Autodesk Inventor part; units mm, degrees
ref_plane "YZ Plane" through (0, 0, 0) normal (1, 0, 0) x (0, 1, 0)
ref_plane "XZ Plane" through (0, 0, 0) normal (0, 1, 0) x (-1, 0, 0)
ref_plane "XY Plane" through (0, 0, 0) normal (0, 0, 1) x (1, 0, 0)
sketch "Skizze1" plane through (0, 0, 0) normal (0, 0, 1) x (1, 0, 0)
  circle A0 centre (0, 0) radius 20
  dimension "d0" = 40
extrude "Extrusion1" add sketch "Skizze1" along normal blind 1
sketch "Skizze2" plane through (0, 0, 1) normal (0, 0, 1) x (1, 0, 0)
  circle A0 centre (0, 0) radius 20
  circle A1 centre (0, 0) radius 17
  dimension "d3" = 34
extrude "Extrusion2" add sketch "Skizze2" along normal blind 10 contours A1
sketch "Skizze3" plane through (0, 0, 11) normal (0, 0, 1) x (1, 0, 0)
  circle A0 centre (0, 0) radius 17
  circle A1 centre (0, 0) radius 20
  dimension "d6" = 40
extrude "Extrusion3" add sketch "Skizze3" along normal blind 1 contours A0 | A1
sketch "Skizze6" plane through (0, 0, 12) normal (0, 0, 1) x (1, 0, 0)
  circle A0 centre (0, 0) radius 20
  circle A1 centre (0, 0) radius 5.1
  dimension "d16" = 10.2
extrude "Extrusion6" cut sketch "Skizze6" against normal through all contours A1
properties part number "Motorstange" material "PC/ABS-Kunststoff"
Model file for the job. Use its own axes, mm. A direction names the side the tool comes from. Coordinates: 2 decimals unless noted, no trailing zeros. Loops run counter-clockwise (first coordinate to the right, second up) from the corner with the lowest first, then second, coordinate; pieces in that order, holes last. Notation, with made-up numbers: (-6.5, 15) -> (36.5, 15) arc R25 cw to (36.5, 42) -> close; hole circle Ø1 at (14, 77). An arc over 180 degrees is marked (long way). Answer as a JSON object with one key per item and string values.
Q1. Cut at C-C (y = 15). List the corners of the cut face in (x, z), and give its area (3 significant figures).
Report:
{"outline": "(-13.23, 0) -> (13.23, 0) -> (13.23, 1) -> (8, 1) -> (8, 11) -> (13.23, 11) -> (13.23, 12) -> (-13.23, 12) -> (-13.23, 11) -> (-8, 11) -> (-8, 1) -> (-13.23, 1) -> close", "area": "213 mm2"}
Q2. 3-axis set-ups, long thin cutter, end or side, ignore diameter. For faces 1 (the cylindrical face through (-4.336, 19.524, 0.493)), 2 (the flat face through (-9, -15, 1)): which of +Z, -Z, +X, -X, +Y, -Y reach the whole face in a straight line?
Report:
{"face 1": "+Z, -Z", "face 2": "none"}
Q3. Flat gauge pin, fed straight in: P1, Ø6, axis at x = -2.5, z = 7.5, coming from the +Y side. Where does the tip first touch, or does it go through?
Report:
{"P1": "stops at y = 17"}
Q4. Pull direction Z, two halves, no side cores. Call faces 3 (the cylindrical face through (2.4, -4.5, 6.1)), 4 (the cylindrical face through (9.139, -14.334, 5.93)), 5 (the flat face through (4, -4, 12)): released by +Z, released by -Z, zero draft, split by the parting line, or undercut.
Report:
{"face 3": "zero draft", "face 4": "undercut", "face 5": "released by +Z"}
Q5. Probe probe 1 along Y at (x, z) = (0, 9.75); probe 2 along Z at (x, y) = (15, 10); probe 3 along Y at (x, z) = (3, 9.5). List the from-to ranges inside material, lowest first.
Report:
{"probe 1": "y = -17 to -5.1, 5.1 to 17", "probe 2": "z = 0 to 1, 11 to 12", "probe 3": "y = -16.73 to -4.12, 4.12 to 16.73"}
Q6. Cut at A-A (x = 0). List the corners of the cut face in (y, z).
Report:
{"outline": "(-20, 0) -> (-5.1, 0) -> (-5.1, 12) -> (-20, 12) -> (-20, 11) -> (-17, 11) -> (-17, 1) -> (-20, 1) -> close; (5.1, 0) -> (20, 0) -> (20, 1) -> (17, 1) -> (17, 11) -> (20, 11) -> (20, 12) -> (5.1, 12) -> close"}
Q7. Cut at D-D (z = 7.75). List the corners of the cut face in (x, y), and give its area (3 significant figures).
Report:
{"outline": "circle Ø34 at (0, 0); hole circle Ø10.2 at (0, 0)", "area": "826 mm2"}
